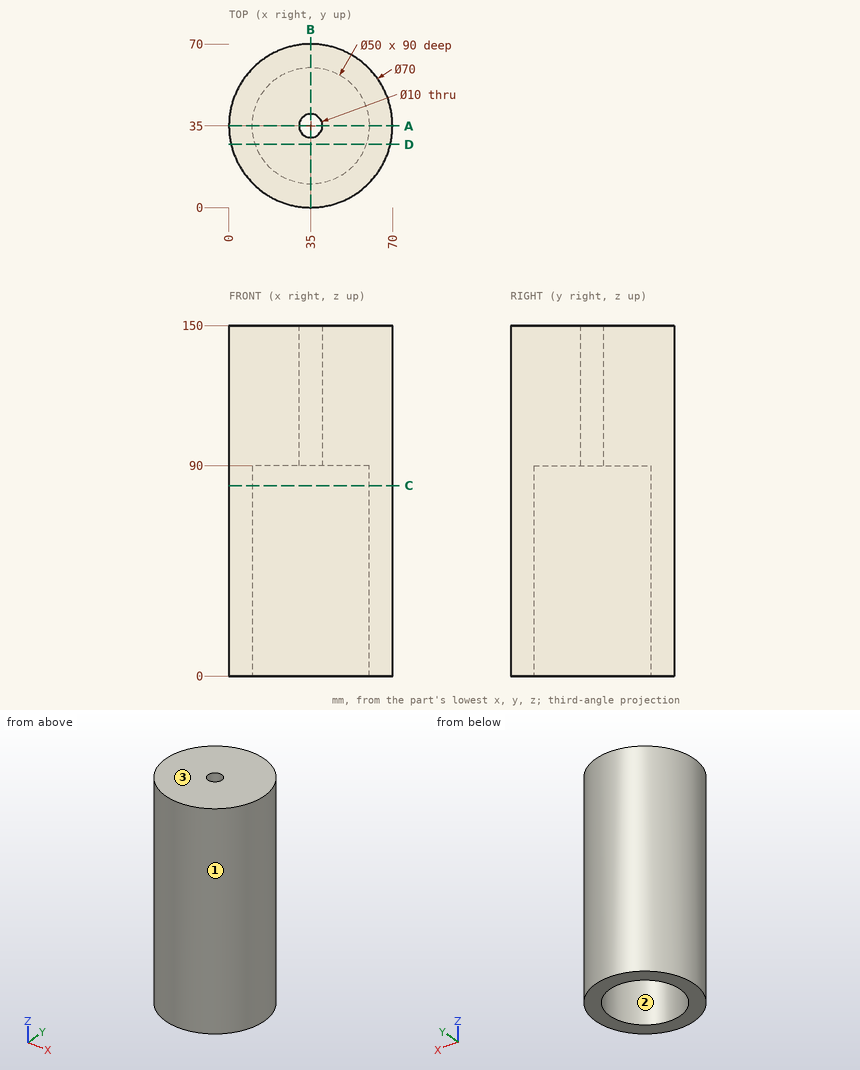
Design review of the part shown in the three views and the two pictorial views. Dimensions are in mm from the part's minimum x, y and z. Give positions to 0.01 mm unless a question says otherwise; leave off trailing zeros. Loops run counter-clockwise (first coordinate to the right, second up) from the corner with the lowest first, then second, coordinate; pieces in that order, holes last. Notation, with made-up numbers: M 44,-9 L 103,-9 A27 cw 103,13 Z; hole C 24,15.5 d1. An arc over 180 degrees is marked long. Answer as a JSON object with one key per item and string values.
Item 1: We need section C-C (z = 81.5). State the section outline as (x, y) points.
Output values:
{"outline": "C 35,35 d70; hole C 35,35 d50"}
Item 2: Mouldability with a two-part tool opening along Y and no side actions: class the marked faces 1, 2 and 3 as pulls with the +Y half, pulls with the -Y half, needs draft (parallel to the pull), parting line crosses it, or undercut.
Output values:
{"face 1": "parting line crosses it", "face 2": "undercut", "face 3": "needs draft"}
Item 3: Wall thickness on line 1 along Y through (x, z) = (35, 70); line 2 along Y through (x, z) = (35, 114); line 3 along Z through (x, y) = (43.5, 19): over which ranges is each line inside the solid? List them lowest first.
Output values:
{"line 1": "y = 0 to 10, 60 to 70", "line 2": "y = 0 to 30, 40 to 70", "line 3": "z = 90 to 150"}
Item 4: We need section A-A (y = 35). State the section outline as (x, z) points, and give its area (3 significant figures).
Output values:
{"outline": "M 0,0 L 10,0 L 10,90 L 30,90 L 30,150 L 0,150 Z; M 40,90 L 60,90 L 60,0 L 70,0 L 70,150 L 40,150 Z", "area": "5,400 mm2"}
Item 5: We need section D-D (y = 27). State the section outline as (x, z) points, and give its area (3 significant figures).
Output values:
{"outline": "M 0.93,0 L 11.31,0 L 11.31,90 L 58.69,90 L 58.69,0 L 69.07,0 L 69.07,150 L 0.93,150 Z", "area": "5,960 mm2"}
Item 6: For P1, Ø4, axis at x = 61.5, z = 108, coming from the -Y side (3 decimals); P2, Ø6, axis at x = 35, y = 35, coming from the -Z side; P3, Ø1, axis at y = 13.5, z = 82.5, coming from the -X side; P4, Ø12, axis at y = 57, z = 64, coming from the -X side, all flat-tipped, find the tip position at first contact; note any pin that passes through.
Output values:
{"P1": "stops at y = 10.005", "P2": "passes through", "P3": "stops at x = 7", "P4": "stops at x = 3.87"}
